Source: three-view drawing plus pictorial views. Frame: mm from the lowest corner of the part. A direction names the side the tool comes from. Coordinates: 2 decimals unless noted, no trailing zeros. Order: outer loops, then holes, each group sorted by start corner. A loop starts at its lowest first (then second) coordinate and runs counter-clockwise, first axis right, second up. Notation, with made-up numbers: (11, -31.75) -> (38, -31.75) arc R16 ccw to (38, -23.75) -> close; hole circle Ø5 at (-20.5, 16.25). An arc over 180 degrees is marked (long way). Use one line per item in the form item = value. Start each with the question number.
1) Section query B-B on y = 18.5. Output: boundary loops of the cut face in (x, z).
2) Section query A-A on x = 18.5. Output: boundary loops of the cut face in (y, z), then the cut area to 3 significant figures.
3) Section query D-D on y = 30. Output: boundary loops of the cut face in (x, z).
4) Access query for the marked faces 1, 2 and 3. Directions: +Z, -Z, +X, -X, +Y, -Y. A direction counts if a zero-diameter tool reaches every point of the face in a straight line with its end or side. Return the directions, or none.
5) Pin query (flat end, axial travel): pin 1 (12 mm diameter, centred on y = 18, z = 21, fed in from +X); pin 2 (3.5 mm diameter, centred on x = 19, y = 3, fed in from +Z); pin 3 (2.5 mm diameter, centred on x = 5.08, y = 26.25, fed in from +Z). Return the tip coordinate at first contact, or that it passes through.
6) Ray query, line 1 along Y through (x, z) = (18.5, 55.1); line 2 along Z through (x, y) = (13.5, 20.5); line 3 along X through (y, z) = (26, 55) (1 decimal). Return the intervals inside material, ascending.
7) Section query C-C on z = 18. Output: boundary loops of the cut face in (x, y), then the cut area to 3 significant figures.
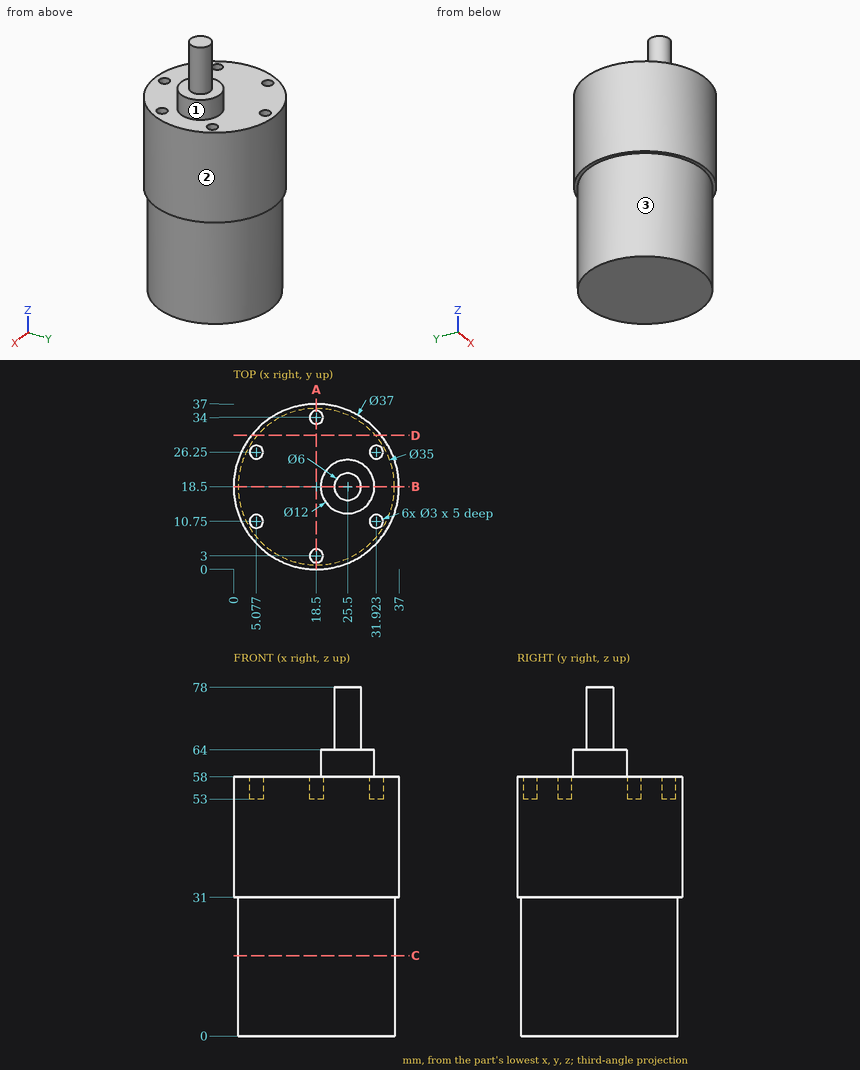
Answers below:
q1.outline = (0, 31) -> (1, 31) -> (1, 0) -> (36, 0) -> (36, 31) -> (37, 31) -> (37, 58) -> (31.5, 58) -> (31.5, 64) -> (28.5, 64) -> (28.5, 78) -> (22.5, 78) -> (22.5, 64) -> (19.5, 64) -> (19.5, 58) -> (0, 58) -> close
q2.outline = (0, 31) -> (1, 31) -> (1, 0) -> (36, 0) -> (36, 31) -> (37, 31) -> (37, 58) -> (35.5, 58) -> (35.5, 53) -> (32.5, 53) -> (32.5, 58) -> (4.5, 58) -> (4.5, 53) -> (1.5, 53) -> (1.5, 58) -> (0, 58) -> close
q2.area = 2,050 mm^2
q3.outline = (4.01, 31) -> (5.31, 31) -> (5.31, 0) -> (31.69, 0) -> (31.69, 31) -> (32.99, 31) -> (32.99, 58) -> (4.01, 58) -> close
q4.face_1 = +Z
q4.face_2 = +Z, -Z
q4.face_3 = -Z
q5.pin_1 = 36
q5.pin_2 = 58
q5.pin_3 = 53
q6.line_1 = 0 to 1.5, 4.5 to 32.5, 35.5 to 37
q6.line_2 = 0 to 58
q6.line_3 = 1.6 to 3.6, 6.6 to 30.4, 33.4 to 35.4
q7.outline = circle Ø35 at (18.5, 18.5)
q7.area = 962 mm^2
